Here's the drawing with two shaded views (mm, measured from the low corner). I have some questions. Give positions to 0.01 mm unless a question says otherwise; leave off trailing zeros. Loops run counter-clockwise (first coordinate to the right, second up) from the corner with the lowest first, then second, coordinate; pieces in that order, holes last. Notation, with made-up numbers: (81, 77) -> (129, 77) arc R21 cw to (129, 107) -> close; hole circle Ø4 at (-22, 71). An arc over 180 degrees is marked (long way). Answer in a Markdown table with one row per item. Add a question column.
Item 1: If we section it at A-A (z = 51): Write out the boundary of the cut face in (x, y), then the cut area to 3 significant figures.
Item 2: If we section it at C-C (y = 2.1): Give the number of separate pieces and of enclosed holes in the cut face, then the cut area to 3 significant figures.
Item 3: If we section it at B-B (x = 87.5): Write out the boundary of the cut face in (y, z).
Item 4: For P1, Ø1.2, axis at x = 8.5, y = 1.5, coming from the -Z side; P2, Ø2, axis at x = 67.5, y = 3.5, coming from the +Z side; P3, Ø2, axis at x = 19.5, y = 2, coming from the -Z side; P4, Ø1.2, axis at x = 48.5, y = 2, coming from the -Z side, each with a flat end and sliding along its axis, tell me the tip position at first contact or that it passes through.
Item 5: If we section it at D-D (x = 27.5): Write out the boundary of the cut face in (y, z), then the cut area to 3 significant figures.
Item 6: If I drill on line 1 (X direction, y = 0.3, z = 9); line 2 (X direction, y = 2.2, z = 55); line 3 (X direction, y = 1.9, z = 41.5), over which ranges is the centre line in solid material (lowest first)?
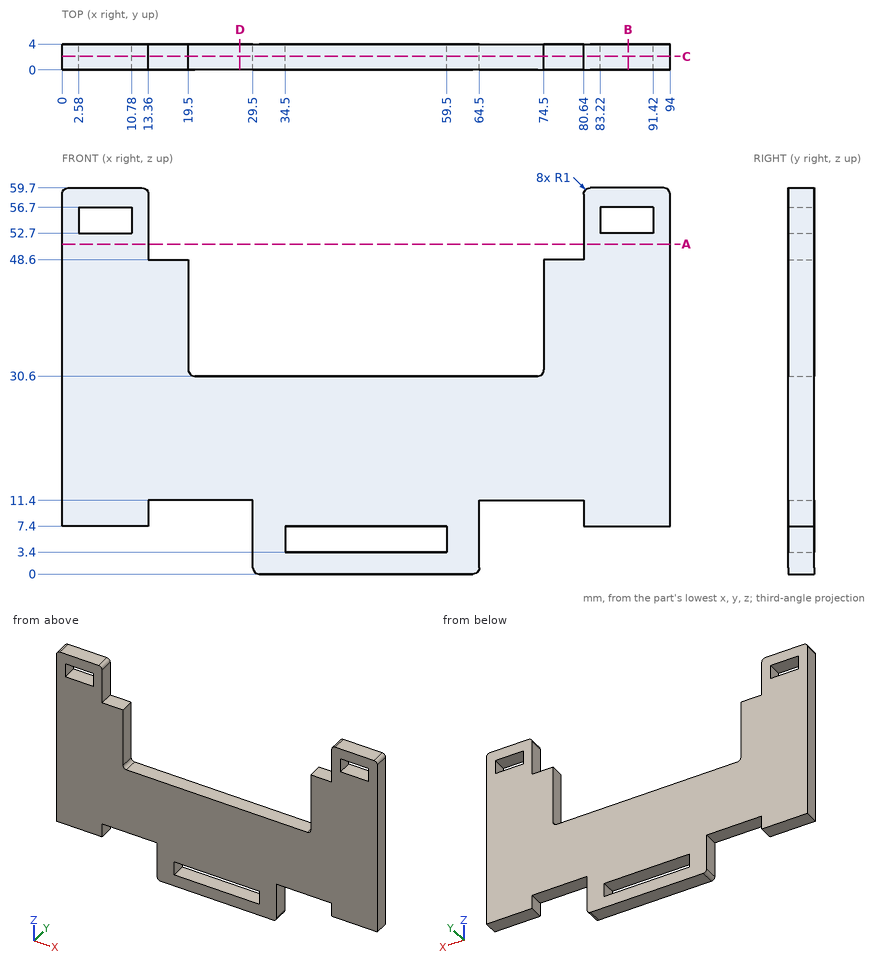
Recorded:
| question | item | result |
|---|---|---|
| 1 | outline | (0, 0) -> (13.36, 0) -> (13.36, 4) -> (0, 4) -> close; (80.64, 0) -> (94, 0) -> (94, 4) -> (80.64, 4) -> close |
| 1 | area | 107 mm^2 |
| 2 | separate pieces | 1 |
| 2 | enclosed holes | 3 |
| 2 | area | 3,140 mm^2 |
| 3 | outline | (0, 7.4) -> (4, 7.4) -> (4, 52.7) -> (0, 52.7) -> close; (0, 56.7) -> (4, 56.7) -> (4, 59.7) -> (0, 59.7) -> close |
| 4 | P1 | stops at z = 7.4 |
| 4 | P2 | stops at z = 30.6 |
| 4 | P3 | stops at z = 11.4 |
| 4 | P4 | stops at z = 0 |
| 5 | outline | (0, 11.4) -> (4, 11.4) -> (4, 30.6) -> (0, 30.6) -> close |
| 5 | area | 76.8 mm^2 |
| 6 | line 1 | x = 0 to 13.36, 29.5 to 64.5, 80.64 to 94 |
| 6 | line 2 | x = 0 to 2.58, 10.78 to 13.36, 80.64 to 83.22, 91.42 to 94 |
| 6 | line 3 | x = 0 to 19.5, 74.5 to 94 |
